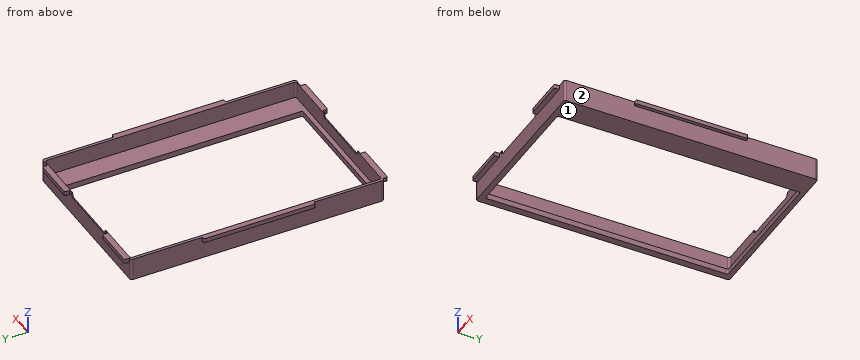
from build123d import *

# Parameters (mm, degrees)
BOX011_W      = 4
BOX011_H      = 80
BOX011_DEPTH  = 3
FILLET006_R   = 1
BOX010_W      = 30
BOX010_H      = 4
BOX010_DEPTH  = 3
FILLET007_R   = 1
BOX009_W      = 30
BOX009_H      = 4
BOX009_DEPTH  = 3
FILLET008_R   = 1
BOX008_W      = 30
BOX008_H      = 4
BOX008_DEPTH  = 3
FILLET009_R   = 1
BOX013_W      = 4
BOX013_H      = 80
BOX013_DEPTH  = 3
FILLET010_R   = 1
BOX012_W      = 30
BOX012_H      = 4
BOX012_DEPTH  = 3
FILLET005_R   = 1
BOX006_W      = 45
BOX006_H      = 10
BOX006_DEPTH  = 10
BOX007_W      = 45
BOX007_H      = 10
BOX007_DEPTH  = 10
FILLET004_1_R = 2
FILLET004_2_R = 1
BOX003_W      = 116
BOX003_H      = 179.5
BOX003_DEPTH  = 20
FILLET002_R   = 1.5
BOX002_W      = 120
BOX002_H      = 181
BOX002_DEPTH  = 12
FILLET003_R   = 1.5
BOX001_W      = 98
BOX001_H      = 173.5
BOX001_DEPTH  = 4
FILLET_R      = 1.5
BOX_W         = 120
BOX_H         = 181
BOX_DEPTH     = 4
FILLET001_R   = 1.5


with BuildPart() as fillet006:
    # Box011 → Box011 (new body)
    with BuildSketch(Plane(origin=(0, 50, 5), x_dir=(1, 0, 0), z_dir=(0, 0, 1))):
        with Locations((2, 40)):
            Rectangle(BOX011_W, BOX011_H)
    extrude(amount=BOX011_DEPTH)

    # Fillet006
    fillet006_edges = [fillet006.edges().sort_by_distance(p)[0] for p in [
        (0, 50, 6.5),
        (0, 130, 6.5),
    ]]
    fillet(fillet006_edges, radius=FILLET006_R)


with BuildPart() as fillet007:
    # Box010 → Box010 (new body)
    with BuildSketch(Plane(origin=(85, -3.5, 5), x_dir=(1, 0, 0), z_dir=(0, 0, 1))):
        with Locations((15, 2)):
            Rectangle(BOX010_W, BOX010_H)
    extrude(amount=BOX010_DEPTH)

    # Fillet007
    fillet007_edges = [fillet007.edges().sort_by_distance(p)[0] for p in [
        (85, -3.5, 6.5),
        (115, -3.5, 6.5),
    ]]
    fillet(fillet007_edges, radius=FILLET007_R)


with BuildPart() as fillet008:
    # Box009 → Box009 (new body)
    with BuildSketch(Plane(origin=(4, 180.5, 5), x_dir=(1, 0, 0), z_dir=(0, 0, 1))):
        with Locations((15, 2)):
            Rectangle(BOX009_W, BOX009_H)
    extrude(amount=BOX009_DEPTH)

    # Fillet008
    fillet008_edges = [fillet008.edges().sort_by_distance(p)[0] for p in [
        (4, 184.5, 6.5),
        (34, 184.5, 6.5),
    ]]
    fillet(fillet008_edges, radius=FILLET008_R)


with BuildPart() as fillet009:
    # Box008 → Box008 (new body)
    with BuildSketch(Plane(origin=(85, 180.5, 5), x_dir=(1, 0, 0), z_dir=(0, 0, 1))):
        with Locations((15, 2)):
            Rectangle(BOX008_W, BOX008_H)
    extrude(amount=BOX008_DEPTH)

    # Fillet009
    fillet009_edges = [fillet009.edges().sort_by_distance(p)[0] for p in [
        (85, 184.5, 6.5),
        (115, 184.5, 6.5),
    ]]
    fillet(fillet009_edges, radius=FILLET009_R)


with BuildPart() as fillet010:
    # Box013 → Box013 (new body)
    with BuildSketch(Plane(origin=(120.5, 50, 5), x_dir=(1, 0, 0), z_dir=(0, 0, 1))):
        with Locations((2, 40)):
            Rectangle(BOX013_W, BOX013_H)
    extrude(amount=BOX013_DEPTH)

    # Fillet010
    fillet010_edges = [fillet010.edges().sort_by_distance(p)[0] for p in [
        (124.5, 50, 6.5),
        (124.5, 130, 6.5),
    ]]
    fillet(fillet010_edges, radius=FILLET010_R)


with BuildPart() as fusion002:
    # Box012 → Box012 (new body)
    with BuildSketch(Plane(origin=(4, -3.5, 5), x_dir=(1, 0, 0), z_dir=(0, 0, 1))):
        with Locations((15, 2)):
            Rectangle(BOX012_W, BOX012_H)
    extrude(amount=BOX012_DEPTH)

    # Fillet005
    fillet005_edges = [fusion002.edges().sort_by_distance(p)[0] for p in [
        (4, -3.5, 6.5),
        (34, -3.5, 6.5),
    ]]
    fillet(fillet005_edges, radius=FILLET005_R)

    # Fusion002: union Fillet006, Fillet007, Fillet008, Fillet009, Fillet010
    add(fillet006.part)
    add(fillet007.part)
    add(fillet008.part)
    add(fillet009.part)
    add(fillet010.part)


with BuildPart() as fusion002_1:
    # Fusion002 placement: moved
    add(fusion002.part.moved(Location((0, 0, 8))))


with BuildPart() as cube006:
    # Box006 → Box006 (new body)
    with BuildSketch(Plane(origin=(15, -5, 0), x_dir=(1, 0, 0), z_dir=(0, 0, 1))):
        with Locations((22.5, 5)):
            Rectangle(BOX006_W, BOX006_H)
    extrude(amount=BOX006_DEPTH)


with BuildPart() as fillet004:
    # Box007 → Box007 (new body)
    with BuildSketch(Plane(origin=(15, 175, 0), x_dir=(1, 0, 0), z_dir=(0, 0, 1))):
        with Locations((22.5, 5)):
            Rectangle(BOX007_W, BOX007_H)
    extrude(amount=BOX007_DEPTH)

    # Fusion: union Cube006
    add(cube006.part)


with BuildPart() as fillet004_1:
    # Fusion placement: moved
    add(fillet004.part.moved(Location((22, 0, 13))))

    # Fillet004 1
    fillet004_1_edges = [fillet004_1.edges().sort_by_distance(p)[0] for p in [
        (37, 180, 13),
        (82, 180, 13),
    ]]
    fillet(fillet004_1_edges, radius=FILLET004_1_R)

    # Fillet004 2
    fillet004_2_edges = [fillet004_1.edges().sort_by_distance(p)[0] for p in [
        (37, 0, 13),
        (82, 0, 13),
    ]]
    fillet(fillet004_2_edges, radius=FILLET004_2_R)


with BuildPart() as fillet002:
    # Box003 → Box003 (new body)
    with BuildSketch(Plane(origin=(4, 0.75, 4), x_dir=(1, 0, 0), z_dir=(0, 0, 1))):
        with Locations((58, 89.75)):
            Rectangle(BOX003_W, BOX003_H)
    extrude(amount=BOX003_DEPTH)

    # Fillet002
    fillet002_edges = [fillet002.edges().sort_by_distance(p)[0] for p in [
        (4, 0.75, 14),
        (4, 180.25, 14),
        (120, 0.75, 14),
        (120, 180.25, 14),
    ]]
    fillet(fillet002_edges, radius=FILLET002_R)


with BuildPart() as cut002:
    # Box002 → Box002 (new body)
    with BuildSketch(Plane(origin=(2, 0, 4), x_dir=(1, 0, 0), z_dir=(0, 0, 1))):
        with Locations((60, 90.5)):
            Rectangle(BOX002_W, BOX002_H)
    extrude(amount=BOX002_DEPTH)

    # Fillet003
    fillet003_edges = [cut002.edges().sort_by_distance(p)[0] for p in [
        (2, 0, 10),
        (2, 181, 10),
        (122, 0, 10),
        (122, 181, 10),
    ]]
    fillet(fillet003_edges, radius=FILLET003_R)

    # Cut001: cut Fillet002
    add(fillet002.part, mode=Mode.SUBTRACT)

    # Cut002: cut Fillet004
    add(fillet004_1.part, mode=Mode.SUBTRACT)


with BuildPart() as fillet_body:
    # Box001 → Box001 (new body)
    with BuildSketch(Plane(origin=(7, 4, 0), x_dir=(1, 0, 0), z_dir=(0, 0, 1))):
        with Locations((49, 86.75)):
            Rectangle(BOX001_W, BOX001_H)
    extrude(amount=BOX001_DEPTH)

    # Fillet
    fillet_edges = [fillet_body.edges().sort_by_distance(p)[0] for p in [
        (7, 4, 2),
        (7, 177.5, 2),
        (105, 4, 2),
        (105, 177.5, 2),
    ]]
    fillet(fillet_edges, radius=FILLET_R)


with BuildPart() as fusion003:
    # Box → Box (new body)
    with BuildSketch(Plane(origin=(2, 0, 0), x_dir=(1, 0, 0), z_dir=(0, 0, 1))):
        with Locations((60, 90.5)):
            Rectangle(BOX_W, BOX_H)
    extrude(amount=BOX_DEPTH)

    # Fillet001
    fillet001_edges = [fusion003.edges().sort_by_distance(p)[0] for p in [
        (2, 0, 2),
        (2, 181, 2),
        (122, 0, 2),
        (122, 181, 2),
    ]]
    fillet(fillet001_edges, radius=FILLET001_R)

    # Cut: cut Fillet body
    add(fillet_body.part, mode=Mode.SUBTRACT)

    # Fusion001: union Cut002
    add(cut002.part)

    # Fusion003: union Fusion002
    add(fusion002_1.part)


solid = fusion003.part
The listing builds one solid part. Answer for the finished solid, in the listing's coordinates (mm). Face numbers are marked on the shaded views. Round coordinates to 2 decimals unless told otherwise and drop trailing zeros. Order: outer loops, then holes, each group sorted by start corner. A loop starts at its lowest first (then second) coordinate and runs counter-clockwise, first axis right, second up. Notation, with made-up numbers: M 15.25,-13 L 74.25,-13 A17 cw 74.25,-3 Z; hole C 37,84.25 d2. An arc over 180 degrees is marked long. Answer in a Markdown table with one row per item. Add a question column.
1) The part is cut by section C-C on z = 8.25. Determine the outline of the cut face in (x, y), plus the area to 3 significant figures.
2) The part is cut by section B-B on y = 90. Determine the outline of the cut face in (x, z).
3) Flat-ended cylindrical pins translate along their axes: pin 1 Ø3 at (y, z) = (-2, 14) entering from -X; pin 2 Ø1.5 at (x, z) = (13.5, 2) entering from +Y; pin 3 Ø3 at (x, y) = (110, 76.5) entering from +Z. Find the tip coordinate at first contact, or state that the pin passes through.
4) The part is cut by section A-A on x = 93.5. Determine the outline of the cut face in (y, z), plus the area to 3 significant figures.
5) Determine the mould class of the marked faces 1 and 2 for opening direction Z: pulls with the +Z half, pulls with the -Z half, needs draft (parallel to the pull), parting line crosses it, or undercut.
6) The part is cut by section D-D on y = 17. Determine the outline of the cut face in (x, z).
7) Consider line 1 along Y through (x, z) = (51, 10.5); line 2 along X through (y, z) = (127, 3.25); line 3 along Y through (x, z) = (102.5, 3). Determine where each line is inside the solid, lowest interval first. Write a range as from..to.
Findings below:
| question | item | result |
|---|---|---|
| 1 | outline | M 2,1.5 A1.5 ccw 3.5,0 L 120.5,0 A1.5 ccw 122,1.5 L 122,179.5 A1.5 ccw 120.5,181 L 3.5,181 A1.5 ccw 2,179.5 Z; hole M 4,2.25 A1.5 ccw 5.5,0.75 L 118.5,0.75 A1.5 ccw 120,2.25 L 120,178.75 A1.5 ccw 118.5,180.25 L 5.5,180.25 A1.5 ccw 4,178.75 Z |
| 1 | area | 898 mm² |
| 2 | outline | M 0,13 L 2,13 L 2,0 L 7,0 L 7,4 L 4,4 L 4,16 L 0,16 Z; M 105,0 L 122,0 L 122,13 L 124.5,13 L 124.5,16 L 120,16 L 120,4 L 105,4 Z |
| 3 | pin 1 | stops at x = 4 |
| 3 | pin 2 | stops at y = 181 |
| 3 | pin 3 | stops at z = 4 |
| 4 | outline | M -3.5,13 L 0,13 L 0,0 L 4,0 L 4,4 L 0.75,4 L 0.75,16 L -3.5,16 Z; M 177.5,0 L 181,0 L 181,13 L 184.5,13 L 184.5,16 L 180.25,16 L 180.25,4 L 177.5,4 Z |
| 4 | area | 69.0 mm² |
| 5 | face 1 | pulls with the -Z half |
| 5 | face 2 | needs draft |
| 6 | outline | M 2,0 L 7,0 L 7,4 L 4,4 L 4,16 L 2,16 Z; M 105,0 L 122,0 L 122,16 L 120,16 L 120,4 L 105,4 Z |
| 7 | line 1 | y = 0..0.75, 180.25..181 |
| 7 | line 2 | x = 2..7, 105..122 |
| 7 | line 3 | y = 0..4, 177.5..181 |
